from build123d import *

# Parameters (mm, degrees)
SKETCH1_W           = 50.8
SKETCH1_H           = 304.8
BOSS_EXTRUDE1_DEPTH = 6.35
SKETCH2_R           = 4.1021
SKETCH2_R_2         = 2.15265
CUT_EXTRUDE1_DEPTH  = 155.632604906


with BuildPart() as part:
    # Sketch1 → Boss-Extrude1 (new body)
    with BuildSketch(Plane(origin=(0, 0, 0), x_dir=(0, 0, -1), z_dir=(1, 0, 0))):
        Rectangle(SKETCH1_W, SKETCH1_H)
    extrude(amount=-BOSS_EXTRUDE1_DEPTH)

    # Sketch2 → Cut-Extrude1 (cut, through all)
    with BuildSketch(Plane(origin=(0, 0, 0), x_dir=(0, 0, -1), z_dir=(1, 0, 0))):
        with Locations((-12.7, -95.25)):
            Circle(SKETCH2_R)
        with Locations((12.7, -95.25)):
            Circle(SKETCH2_R)
        with Locations((12.7, -133.35)):
            Circle(SKETCH2_R)
        with Locations((-12.7, -133.35)):
            Circle(SKETCH2_R)
        with Locations((-19.05, 146.05)):
            Circle(SKETCH2_R_2)
        with Locations((0, 146.05)):
            Circle(SKETCH2_R_2)
        with Locations((19.05, 146.05)):
            Circle(SKETCH2_R_2)
    extrude(amount=-CUT_EXTRUDE1_DEPTH, mode=Mode.SUBTRACT)


solid = part.part
Work out the finished part from the listing and answer in its coordinate system (mm). Round coordinates to 2 decimals unless told otherwise and drop trailing zeros. Order: outer loops, then holes, each group sorted by start corner. A loop starts at its lowest first (then second) coordinate and runs counter-clockwise, first axis right, second up. Notation, with made-up numbers: M 29,37.5 L 47,37.5 A13 ccw 47,46.5 Z; hole C -5,-11 d7. An arc over 180 degrees is marked long. Put each result on its own line as item: value. Start each with the question number.
Q1. Section B-B, the plane z = 12.7 is taken. Write down the section's boundary in (x, y), and give its area (3 significant figures).
Q2. For a pull along Z with two mould halves and no side action, classify faces 1 (the flat face through (-3, -2, 25.4)), 2 (the flat face through (-3, 152.4, 0)), 3 (the flat face through (-3, -2, -25.4)), 4 (the cylindrical face through (-3.131, -91.183, 13.234)) as pulls with the +Z half, pulls with the -Z half, needs draft (parallel to the pull), parting line crosses it, or undercut.
Q3. Section C-C, the plane x = -2.25 is taken. Write down the section's boundary in (y, z), and give its area (3 significant figures).
Q4. Straight lines are drawn through the part: L1, parallel to Y at x = -4.5, z = -12.7; L2, parallel to Z at x = -5, y = 146.05; L3, parallel to Z at x = -1.25, y = -136.5. For each, find the intervals that lie inside material, in ascending order. Write a range as [from, to].
Q5. Section A-A, the plane y = -133.35 is taken. Write down the section's boundary in (x, z).
Findings below:
1. outline: M -6.35,-152.4 L 0,-152.4 L 0,-137.45 L -6.35,-137.45 Z; M -6.35,-129.25 L 0,-129.25 L 0,-99.35 L -6.35,-99.35 Z; M -6.35,-91.15 L 0,-91.15 L 0,152.4 L -6.35,152.4 Z
1. area: 1,830 mm^2
2. face 1: pulls with the +Z half
2. face 2: needs draft
2. face 3: pulls with the -Z half
2. face 4: undercut
3. outline: M -152.4,-25.4 L 152.4,-25.4 L 152.4,25.4 L -152.4,25.4 Z; hole C -133.35,-12.7 d8.2; hole C -133.35,12.7 d8.2; hole C -95.25,-12.7 d8.2; hole C -95.25,12.7 d8.2; hole C 146.05,-19.05 d4.31; hole C 146.05,0 d4.31; hole C 146.05,19.05 d4.31
3. area: 15,200 mm^2
4. L1: y = [-152.4, -137.45], [-129.25, -99.35], [-91.15, 152.4]
4. L2: z = [-25.4, -21.2], [-16.9, -2.15], [2.15, 16.9], [21.2, 25.4]
4. L3: z = [-25.4, -15.33], [-10.07, 10.07], [15.33, 25.4]
5. outline: M -6.35,-25.4 L 0,-25.4 L 0,-16.8 L -6.35,-16.8 Z; M -6.35,-8.6 L 0,-8.6 L 0,8.6 L -6.35,8.6 Z; M -6.35,16.8 L 0,16.8 L 0,25.4 L -6.35,25.4 Z
